Read the model definition and answer for the solid it produces. Units are mm, in the model's axes. Face numbers are marked on the shaded views. A direction names the side the tool comes from. Coordinates: 2 decimals unless noted, no trailing zeros. Loops run counter-clockwise (first coordinate to the right, second up) from the corner with the lowest first, then second, coordinate; pieces in that order, holes last. Notation, with made-up numbers: M -27.5,62.25 L -2.5,62.25 A11 cw -2.5,67.25 Z; hole C 35.25,86.5 d2. An arc over 180 degrees is marked long. One line per item, written item: value. Start each with the question number.
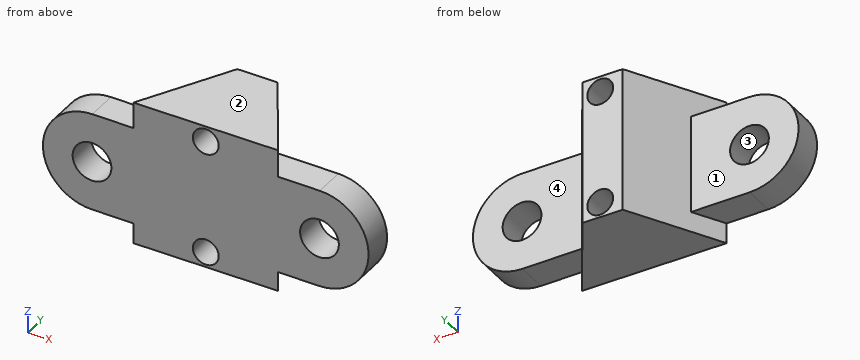
```python
from build123d import *

# Parameters (mm, degrees)
EXTRUDE_1_DEPTH     = 56
SKETCH_3_R          = 7.5
EXTRUDE_3_DEPTH     = 12
SKETCH_4_R          = 5
CUT_EXTRUDE_1_DEPTH = 92.268833673


with BuildPart() as part:
    # 스케치1 → 보스-돌출1 (new body)
    with BuildSketch(Plane.XY):
        Polygon((-28, 0), (28, 0), (6.865874615, 35), (-8.698826384, 35), align=None)
    extrude(amount=EXTRUDE_1_DEPTH)

    # 스케치3 → 보스-돌출3 (add)
    with BuildSketch(Plane.XZ):
        with BuildLine():
            Line((-43.863739751, 45.99090258), (44.136260249, 45.35978625))
            ThreePointArc((44.136260249, 45.35978625), (62.999511392, 26.224014609), (43.863739751, 7.360763465))
            Line((43.863739751, 7.360763465), (-44.136260249, 7.991879796))
            ThreePointArc((-44.136260249, 7.991879796), (-62.999511392, 27.127651437), (-43.863739751, 45.99090258))
        make_face()
        with Locations(Location((-44, 26.991391188, 0), (0, 0, 270))):
            Circle(SKETCH_3_R, mode=Mode.SUBTRACT)
        with Locations(Location((44, 26.360274858, 0), (0, 0, 270))):
            Circle(SKETCH_3_R, mode=Mode.SUBTRACT)
    extrude(amount=-EXTRUDE_3_DEPTH)

    # 스케치4 → 컷-돌출1 (cut, through all)
    with BuildSketch(Plane(origin=(0, 35, 0), x_dir=(1, 0, 0), z_dir=(0, 1, 0))):
        with Locations(Location((0, -5.967731641, 0), (0, 0, 270))):
            Circle(SKETCH_4_R)
        with Locations(Location((0, -49.967731641, 0), (0, 0, 270))):
            Circle(SKETCH_4_R)
    extrude(amount=-CUT_EXTRUDE_1_DEPTH, mode=Mode.SUBTRACT)


solid = part.part
```
1) Section C-C (y = 3.5) is taken. Determine the outline of the cut face in (x, z), then the cut area to 3 significant figures.
2) Flat-ended cylindrical pins translate along their axes: pin 1 (8 mm diameter, centred on y = 6.5, z = 40.5, fed in from -X); pin 2 (8 mm diameter, centred on x = 16.5, y = 23, fed in from +Z); pin 3 (6 mm diameter, centred on y = 12.5, z = 12, fed in from -X); pin 4 (1 mm diameter, centred on x = -46, y = 9, fed in from +Z). Find the tip coordinate at first contact, or state that the pin passes through.
3) A tool of negligible diameter and unlimited length cuts with its end or side. For the marked faces 1 and 2, from which of +Z, -Z, +X, -X, +Y, -Y can it reach the whole face along a straight path? Write none if from no direction.
4) For a pull along X with two mould halves and no side action, classify the marked faces 3 and 4 as released by +X, released by -X, zero draft, split by the parting line, or undercut.
5) Section A-A (x = 0) is taken. Determine the outline of the cut face in (y, z).
6) Section B-B (z = 31.5) is taken. Determine the outline of the cut face in (x, y), then the cut area to 3 significant figures.
7) Consider line 1 along Y through (x, z) = (58.5, 31); line 2 along X through (y, z) = (7.5, 46.5); line 3 along X through (y, z) = (2.5, 11.5). Determine where each line is inside the solid, lowest interval first.
8) Section D-D (x = -47.5) is taken. Determine the outline of the cut face in (y, z).
Results found:
1. outline: M -44.14,7.99 L -26.07,7.86 L -26.07,0 L 25.89,0 L 25.89,7.49 L 43.86,7.36 A19 ccw 44.14,45.36 L 25.89,45.49 L 25.89,56 L -26.07,56 L -26.07,45.86 L -43.86,45.99 A19 ccw Z; hole C -44,26.99 d15; hole C 0,5.97 d10; hole C 0,49.97 d10; hole C 44,26.36 d15
1. area: 4,900 mm²
2. pin 1: stops at x = -60.45
2. pin 2: stops at z = 56
2. pin 3: stops at x = -58.7
2. pin 4: stops at z = 45.93
3. face 1: +Z, -Z, -X, +Y
3. face 2: +Z, +X, -X, +Y, -Y
4. face 3: undercut
4. face 4: zero draft
5. outline: M 0,0 L 35,0 L 35,0.97 L 0,0.97 Z; M 0,10.97 L 35,10.97 L 35,44.97 L 0,44.97 Z; M 0,54.97 L 35,54.97 L 35,56 L 0,56 Z
6. outline: M -62.46,0 L -49.99,0 L -49.99,12 L -62.46,12 Z; M -38.01,0 L 38.54,0 L 38.54,12 L 20.75,12 L 6.87,35 L -8.7,35 L -21.38,12 L -38.01,12 Z; M 49.46,0 L 62.29,0 L 62.29,12 L 49.46,12 Z
6. area: 1,890 mm²
7. line 1: y = 0 to 12
7. line 2: x = -23.86 to -3.6, 3.6 to 23.47
7. line 3: x = -55 to 55.84
8. outline: M 0,8.32 L 12,8.32 L 12,20.36 L 0,20.36 Z; M 0,33.62 L 12,33.62 L 12,45.67 L 0,45.67 Z
